from build123d import *

# Parameters (mm, degrees)
BOSS_EXTRUDE1_DEPTH = 84.074
SKETCH3_W           = 76.581
SKETCH3_H           = 76.581
BOSS_EXTRUDE2_DEPTH = 31.75
SKETCH_D_R          = 23.8125
BOSS_EXTRUDE3_DEPTH = 104.902
CUT_EXTRUDE1_DEPTH  = 35.56
FILLET1_R           = 6.35
FILLET2_R           = 1.27
KEYWAY_START        = 16.5989
KEYWAY_DEPTH        = 63.6491
CHAMFER1_SIZE       = 0.381
SKETCH7_R           = 23.8125
CUT_EXTRUDE3_DEPTH  = 221.726


with BuildPart() as part:
    # L,M → Boss-Extrude1 (new body)
    with BuildSketch(Plane.XY):
        Polygon((-100.076, 68.326), (100.076, 68.326), (100.076, 207.077403609), (84.201, 222.952403609), (84.201, 288.603596391), (37.778596391, 335.026), (-37.778596391, 335.026), (-84.201, 288.603596391), (-84.201, 222.952403609), (-100.076, 207.077403609), align=None)
    extrude(amount=BOSS_EXTRUDE1_DEPTH)

    # Sketch3 → Boss-Extrude2 (add)
    with BuildSketch(Plane.XY.offset(84.074)):
        with Locations((0, 255.778)):
            Rectangle(SKETCH3_W, SKETCH3_H)
    extrude(amount=BOSS_EXTRUDE2_DEPTH)

    # D → Boss-Extrude3 (add)
    with BuildSketch(Plane.XY.offset(115.824)):
        with Locations((0, 255.778)):
            Circle(SKETCH_D_R)
    extrude(amount=BOSS_EXTRUDE3_DEPTH)

    # Sketch5 → Cut-Extrude1 (cut)
    with BuildSketch(Plane.XY.offset(84.074)):
        Polygon((100.076, 114.748403609), (53.653596391, 68.326), (100.076, 68.326), align=None)
        Polygon((-100.076, 68.326), (-100.076, 114.748403609), (-53.653596391, 68.326), align=None)
    extrude(amount=-CUT_EXTRUDE1_DEPTH, mode=Mode.SUBTRACT)

    # Fillet1
    fillet1_edges = [part.edges().sort_by_distance(p)[0] for p in [
        (-38.2905, 294.0685, 99.949),
        (-38.2905, 217.4875, 99.949),
        (38.2905, 217.4875, 99.949),
        (38.2905, 294.0685, 99.949),
    ]]
    fillet(fillet1_edges, radius=FILLET1_R)

    # Fillet2
    fillet2_edges = [part.edges().sort_by_distance(p)[0] for p in [
        (100.076, 160.912903609, 84.074),
        (76.864798195, 91.537201805, 84.074),
        (92.1385, 215.014903609, 84.074),
        (84.201, 255.778, 84.074),
        (60.989798195, 311.814798195, 84.074),
        (0, 335.026, 84.074),
        (0, 68.326, 84.074),
        (-60.989798195, 311.814798195, 84.074),
        (-84.201, 255.778, 84.074),
        (-92.1385, 215.014903609, 84.074),
        (-100.076, 160.912903609, 84.074),
        (-76.864798195, 91.537201805, 84.074),
        (0, 217.4875, 84.074),
        (-38.2905, 255.778, 84.074),
        (38.2905, 255.778, 84.074),
        (0, 294.0685, 84.074),
        (-36.430628061, 219.347371939, 84.074),
        (36.430628061, 219.347371939, 84.074),
        (-36.430628061, 292.208628061, 84.074),
        (36.430628061, 292.208628061, 84.074),
    ]]
    fillet(fillet2_edges, radius=FILLET2_R)

    # Sketch6 → Keyway (cut, through all)
    with BuildSketch(Plane(origin=(0, 255.778, 0), x_dir=(-1, 0, 0), z_dir=(0, 1, 0)).offset(KEYWAY_START)):
        with BuildLine():
            Line((6.35, 220.726), (6.35, 141.224))
            ThreePointArc((6.35, 141.224), (0, 134.874), (-6.35, 141.224))
            Line((-6.35, 141.224), (-6.35, 220.726))
            ThreePointArc((-6.35, 220.726), (0, 227.076), (6.35, 220.726))
        make_face()
    extrude(amount=KEYWAY_DEPTH, mode=Mode.SUBTRACT)

    # Chamfer1
    chamfer1_edges = [part.edges().sort_by_distance(p)[0] for p in [
        (-14.419184811, 236.827478487, 220.726),
    ]]
    chamfer(chamfer1_edges, length=CHAMFER1_SIZE)

    # Sketch7 → Cut-Extrude3 (cut, through all)
    with BuildSketch(Plane(origin=(0, 0, 0), x_dir=(-1, 0, 0), z_dir=(0, 0, -1))):
        with Locations((0, 136.652)):
            Circle(SKETCH7_R)
    extrude(amount=-CUT_EXTRUDE3_DEPTH, mode=Mode.SUBTRACT)


solid = part.part
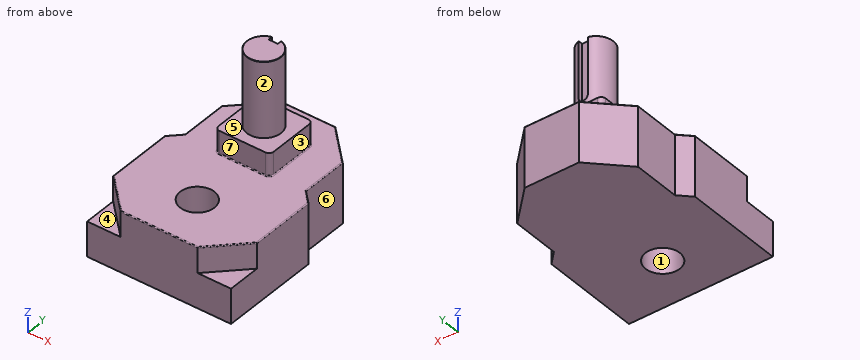
Part model, mm, in its own coordinate system. Face numbers are marked on the shaded views. A direction names the side the tool comes from. Coordinates: 2 decimals unless noted, no trailing zeros. Loops run counter-clockwise (first coordinate to the right, second up) from the corner with the lowest first, then second, coordinate; pieces in that order, holes last. Notation, with made-up numbers: (63.25, -18) -> (95.25, -18) arc R26 ccw to (95.25, -2) -> close; hole circle Ø4 at (-2, -2). An arc over 180 degrees is marked (long way). Use a Markdown table: item, result. Add a question column.
Item 1: Band-saw the part on A-A on x = 0. Write the cut outline in (y, z) (1 decimal), plus the area to 3 significant figures.
Item 2: Pull direction X, two halves, no side cores. Call the marked faces 1, 2, 3 and 4: +X half, -X half, draft (parallel to the pull), parting line (faces both ways), or undercut.
Item 3: Probe probe 1 along Y at (x, z) = (0, 58.5); probe 2 along Z at (x, y) = (37, 164.5); probe 3 along Y at (x, z) = (-15.5, 74). List the from-to ranges inside material, lowest first.
Item 4: Flat gauge pins, fed straight in: P1, Ø23, axis at x = -71, y = 91, coming from the +Z side; P2, Ø6, axis at x = 50.5, y = 264.5, coming from the -Z side; P3, Ø3, axis at y = 275.5, z = 174.5, coming from the -X side; P4, Ø24.5, axis at y = 253, z = 100, coming from the -X side. Where does each tip first touch, or does it go through?
Item 5: Band-saw the part on B-B on z = 95.5. Write the cut outline in (x, y).
Item 6: Which spindle directions (+Z, -Z, +X, -X, +Y, -Y) get a long thin tool onto all of the face, cutting with end or side? Do the marked faces 5, 6 and 7. Say none if no direction does.
Item 7: Band-saw the part on C-C on y = 183. Write the cut outline in (x, z).
Geometry says:
| question | item | result |
|---|---|---|
| 1 | outline | (68.3, 0) -> (112.8, 0) -> (112.8, 84.1) -> (69.6, 84.1) arc R1.3 ccw to (68.3, 82.8) -> close; (160.5, 0) -> (335, 0) -> (335, 82.8) arc R1.3 ccw to (333.8, 84.1) -> (295.3, 84.1) arc R1.3 cw to (294.1, 85.3) -> (294.1, 115.8) -> (279.6, 115.8) -> (279.6, 134.9) -> (272.4, 134.9) -> (272.4, 220.7) -> (232.3, 220.7) -> (232, 220.3) -> (232, 115.8) -> (217.5, 115.8) -> (217.5, 85.3) arc R1.3 cw to (216.2, 84.1) -> (160.5, 84.1) -> close |
| 1 | area | 25,200 mm² |
| 2 | face 1 | undercut |
| 2 | face 2 | parting line |
| 2 | face 3 | +X half |
| 2 | face 4 | draft |
| 3 | probe 1 | 68.33 to 112.84, 160.46 to 335.03 |
| 3 | probe 2 | 0 to 84.07 |
| 3 | probe 3 | 68.33 to 118.57, 154.73 to 335.03 |
| 4 | P1 | z = 84.07 |
| 4 | P2 | z = 0 |
| 4 | P3 | x = -15.33 |
| 4 | P4 | x = -38.29 |
| 5 | outline | (-38.29, 223.84) arc R6.35 ccw to (-31.94, 217.49) -> (31.94, 217.49) arc R6.35 ccw to (38.29, 223.84) -> (38.29, 287.72) arc R6.35 ccw to (31.94, 294.07) -> (-31.94, 294.07) arc R6.35 ccw to (-38.29, 287.72) -> close |
| 6 | face 5 | +Z |
| 6 | face 6 | +Z, -Z, +X, +Y |
| 6 | face 7 | +Z, +X, -X, -Y |
| 7 | outline | (-100.08, 0) -> (100.08, 0) -> (100.08, 82.8) arc R1.27 ccw to (98.81, 84.07) -> (-98.81, 84.07) arc R1.27 ccw to (-100.08, 82.8) -> close |
